Check sheet for the modelled part. Datum: model origin and axes. Units: mm. A direction names the side the tool comes from. Give positions to 0.01 mm unless a question says otherwise; leave off trailing zeros. Order: outer loops, then holes, each group sorted by start corner. A loop starts at its lowest first (then second) coordinate and runs counter-clockwise, first axis right, second up. Notation, with made-up numbers: M 60,5.5 L 102,5.5 A6 cw 102,12.5 Z; hole C 5,57.25 d1. An arc over 180 degrees is marked long. Answer in a Markdown table with one row per item. Add a question column.
from build123d import *

# Parameters (mm, degrees)
SKETCH1_R           = 1.6
SKETCH1_R_2         = 1.5
BOSS_EXTRUDE3_DEPTH = 3.2
LPATTERN2_COUNT     = 2
LPATTERN2_PITCH     = 6.8
SKETCH9_W           = 9.22
SKETCH9_H           = 12
BOSS_EXTRUDE5_DEPTH = 3.7
SKETCH11_W          = 60.430595346
SKETCH11_H          = 12
BOSS_EXTRUDE6_DEPTH = 3.7
LPATTERN3_COUNT     = 2
LPATTERN3_PITCH     = 76
SKETCH13_W          = 112.501798465
SKETCH13_H          = 66
BOSS_EXTRUDE8_DEPTH = 3
SKETCH14_R          = 1.5
CUT_EXTRUDE2_DEPTH  = 4.318
SKETCH22_W          = 5.174861703
SKETCH22_H          = 10.217447179
BOSS_EXTRUDE9_DEPTH = 4.318


with BuildPart() as part:
    # Sketch1 → Boss-Extrude3 (new body)
    with BuildSketch(Plane.XY):
        with BuildLine():
            Line((-103.947681543, 43.894483621), (110.052318457, 43.894483621))
            ThreePointArc((110.052318457, 43.894483621), (112.1736388, 43.015803964), (113.052318457, 40.894483621))
            Line((113.052318457, 40.894483621), (113.052318457, 34.894483621))
            ThreePointArc((113.052318457, 34.894483621), (112.1736388, 32.773163277), (110.052318457, 31.894483621))
            Line((110.052318457, 31.894483621), (-103.947681543, 31.894483621))
            ThreePointArc((-103.947681543, 31.894483621), (-106.069001887, 32.773163277), (-106.947681543, 34.894483621))
            Line((-106.947681543, 34.894483621), (-106.947681543, 40.894483621))
            ThreePointArc((-106.947681543, 40.894483621), (-106.069001887, 43.015803964), (-103.947681543, 43.894483621))
        make_face()
        with Locations((-102.125890736, 37.895486936)):
            Circle(SKETCH1_R, mode=Mode.SUBTRACT)
        with Locations((-102.125890736, 41.895486936)):
            Circle(SKETCH1_R_2, mode=Mode.SUBTRACT)
        with Locations((-102.125890736, 33.895486936)):
            Circle(SKETCH1_R_2, mode=Mode.SUBTRACT)
        with Locations((109.874217574, 37.891839711)):
            Circle(SKETCH1_R_2, mode=Mode.SUBTRACT)
        with Locations((-12.125890736, 37.895486936)):
            Circle(SKETCH1_R_2, mode=Mode.SUBTRACT)
        with Locations((17.874109264, 37.895486936)):
            Circle(SKETCH1_R_2, mode=Mode.SUBTRACT)
    extrude(amount=BOSS_EXTRUDE3_DEPTH)


with BuildPart() as lpattern2_1:
    # LPattern2: pattern copy
    add(part.part.moved(Location(Vector(0, 0, 1) * (1 * LPATTERN2_PITCH))))


with BuildPart() as part_1:
    add(part.part)

    add(lpattern2_1.part)  # Boss-Extrude5 merges LPattern2_1
    # Sketch9 → Boss-Extrude5 (add)
    with BuildSketch(Plane.XY.offset(3.2)):
        with Locations((3.052318457, 37.894483621)):
            Rectangle(SKETCH9_W, SKETCH9_H)
    extrude(amount=BOSS_EXTRUDE5_DEPTH)

    # Sketch11 → Boss-Extrude6 (add)
    with BuildSketch(Plane.XY.offset(3.2)):
        with Locations((61.010147688, 37.894483621)):
            Rectangle(SKETCH11_W, SKETCH11_H)
        Polygon((-79.696539418, 43.894483621), (-79.758832443, 43.894483621), (-79.758832443, 31.894483621), (-23.819696729, 31.894483621), (-23.819696729, 43.894483621), align=None)
    extrude(amount=BOSS_EXTRUDE6_DEPTH)


with BuildPart() as lpattern3_1:
    # LPattern3: pattern copy
    add(part_1.part.moved(Location(Vector(0, 0, 1) * (1 * LPATTERN3_PITCH))))


with BuildPart() as part_2:
    add(part_1.part)

    add(lpattern3_1.part)  # Boss-Extrude8 merges LPattern3_1
    # Sketch13 → Boss-Extrude8 (add)
    with BuildSketch(Plane(origin=(0, 43.894483621, 0), x_dir=(1, 0, 0), z_dir=(0, 1, 0))):
        with Locations((4.548532601, -43)):
            Rectangle(SKETCH13_W, SKETCH13_H)
    extrude(amount=-BOSS_EXTRUDE8_DEPTH)

    # Sketch14 → Cut-Extrude2 (cut)
    with BuildSketch(Plane(origin=(0, 43.894483621, 0), x_dir=(1, 0, 0), z_dir=(0, 1, 0))):
        with Locations(Location((-46.622366631, -15.08, 0), (0, 0, 270))):
            Circle(SKETCH14_R)
        with Locations(Location((55.719431834, -15.08, 0), (0, 0, 270))):
            Circle(SKETCH14_R)
        with Locations(Location((55.719431834, -70.92, 0), (0, 0, 270))):
            Circle(SKETCH14_R)
        with Locations(Location((-46.622366631, -70.92, 0), (0, 0, 270))):
            Circle(SKETCH14_R)
    extrude(amount=-CUT_EXTRUDE2_DEPTH, mode=Mode.SUBTRACT)

    # Sketch22 → Boss-Extrude9 (add)
    with BuildSketch(Plane.XZ.offset(-40.894483621)):
        with Locations((-36.737847825, 70.891276411)):
            Rectangle(SKETCH22_W, SKETCH22_H)
        with Locations((-21.497847826, 70.891276411)):
            Rectangle(SKETCH22_W, SKETCH22_H)
        with Locations((-6.257847826, 70.891276411)):
            Rectangle(SKETCH22_W, SKETCH22_H)
        with Locations((8.982152175, 70.891276411)):
            Rectangle(SKETCH22_W, SKETCH22_H)
        with Locations((24.222152175, 70.891276411)):
            Rectangle(SKETCH22_W, SKETCH22_H)
        with Locations((39.462152175, 70.891276411)):
            Rectangle(SKETCH22_W, SKETCH22_H)
        with Locations((-21.497847826, 15.011276411)):
            Rectangle(SKETCH22_W, SKETCH22_H)
        with Locations((-6.257847826, 15.011276411)):
            Rectangle(SKETCH22_W, SKETCH22_H)
        with Locations((8.982152175, 15.011276411)):
            Rectangle(SKETCH22_W, SKETCH22_H)
        with Locations((24.222152175, 15.011276411)):
            Rectangle(SKETCH22_W, SKETCH22_H)
        with Locations((39.462152175, 15.011276411)):
            Rectangle(SKETCH22_W, SKETCH22_H)
        with Locations((-36.737847825, 15.011276411)):
            Rectangle(SKETCH22_W, SKETCH22_H)
    extrude(amount=BOSS_EXTRUDE9_DEPTH)


solid = part_2.part
Q1. Thickness scan on probe 1 along Z at (x, y) = (-84.5, 33.5); probe 2 along Z at (x, y) = (27, 41.25); probe 3 along Z at (x, y) = (60, 40). Record the ranges inside material, lowest first.
Q2. Go/stop test with flat-tipped pins: pin 1 (1.6 mm diameter, centred on x = 40, z = 13.5, fed in from -Y); pin 2 (4.5 mm diameter, centred on y = 38.5, z = 15.5, fed in from +X); pin 3 (1.5 mm diameter, centred on y = 41.5, z = 63.5, fed in from -X); pin 4 (5 mm diameter, centred on x = -12.13, y = 37.9, fed in from +Z). Record where each tip stops, or that it passes through.
Q3. Tool access check on faces 1 (the flat face through (-34.15, 39, 71)), 2 (the flat face through (9, 39, 20.12)), 3 (the flat face through (102, 38, 6.8)). Record the directions out of +Z, -Z, +X, -X, +Y, -Y that give a thin tool (end or side, any length) a straight path to the whole face; none if there is none.
Q4. Cross-section at A-A (x = -87.5). Record the boundary of the cut face in (y, z).
Q5. Cross-section at B-B (x = -31.5). Record the boundary of the cut face in (y, z), and give its area (3 significant figures).
Q6. Cross-section at C-C (z = 38). Record the boundary of the cut face in (x, y), and give its area (3 significant figures).
Values follow:
| question | item | result |
|---|---|---|
| 1 | probe 1 | 0 to 3.2, 6.8 to 10, 76 to 79.2, 82.8 to 86 |
| 1 | probe 2 | 0 to 3.2, 6.8 to 79.2, 82.8 to 86 |
| 1 | probe 3 | 0 to 10, 76 to 86 |
| 2 | pin 1 | y = 36.58 |
| 2 | pin 2 | x = 42.05 |
| 2 | pin 3 | x = -51.7 |
| 2 | pin 4 | z = 86 |
| 3 | face 1 | -Y |
| 3 | face 2 | +X, -X, -Y |
| 3 | face 3 | +X, +Y, -Y |
| 4 | outline | M 31.89,0 L 43.89,0 L 43.89,3.2 L 31.89,3.2 Z; M 31.89,6.8 L 43.89,6.8 L 43.89,10 L 31.89,10 Z; M 31.89,76 L 43.89,76 L 43.89,79.2 L 31.89,79.2 Z; M 31.89,82.8 L 43.89,82.8 L 43.89,86 L 31.89,86 Z |
| 5 | outline | M 31.89,0 L 43.89,0 L 43.89,86 L 31.89,86 L 31.89,76 L 40.89,76 L 40.89,10 L 31.89,10 Z |
| 5 | area | 438 mm² |
| 6 | outline | M -51.7,40.89 L 60.8,40.89 L 60.8,43.89 L -51.7,43.89 Z |
| 6 | area | 338 mm² |
